```python
from build123d import *
from build123d.topology import SkipClean

# Parameters (mm, degrees)
SKETCH1_R                = 17.928932
BOSS_EXTRUDE1_DEPTH      = 10
SKETCH2_R                = 7.928932
CUT_EXTRUDE1_DEPTH       = 28.256068
BOSS_EXTRUDE2_REACH      = 46.834
BOSS_EXTRUDE2_END_RADIUS = 17.928932
SKETCH4_R                = 5
BOSS_EXTRUDE5_REACH      = 48.578
BOSS_EXTRUDE5_END_RADIUS = 17.928932
SKETCH11_R               = 5
CUT_EXTRUDE5_DEPTH       = 4
CIRPATTERN1_COUNT        = 2
CIRPATTERN1_ANGLE        = 270
SKETCH21_R               = 7.928932
BOSS_EXTRUDE6_DEPTH      = 20
SKETCH22_R               = 7.928932
BOSS_EXTRUDE7_DEPTH      = 20


with BuildPart() as part:
    # Sketch1 → Boss-Extrude1 (new body)
    with BuildSketch(Plane(origin=(0, 0, 0), x_dir=(1, 0, 0), z_dir=(0, 1, 0))):
        with Locations(Location((0, 0, 0), (0, 0, 270))):
            Circle(SKETCH1_R)
    extrude(amount=BOSS_EXTRUDE1_DEPTH)

    # Sketch2 → Cut-Extrude1 (cut, through all)
    with BuildSketch(Plane(origin=(0, 10, 0), x_dir=(1, 0, 0), z_dir=(0, 1, 0))):
        with Locations(Location((0, 0, 0), (0, 0, 270))):
            Circle(SKETCH2_R)
    extrude(amount=-CUT_EXTRUDE1_DEPTH, mode=Mode.SUBTRACT)

    # Boss-Extrude2: up to this cylinder (the profile starts outside it)
    with SkipClean():  # the faces are left unmerged after this step: merging them gives an invalid solid
        boss_extrude2_end = Plane(origin=(0, 5, 0), z_dir=(0, -1, 0)) * Cylinder(BOSS_EXTRUDE2_END_RADIUS, 130.525864, mode=Mode.PRIVATE)
        # Sketch4 → Boss-Extrude2 (add, up to the surface)
        with BuildSketch(Plane(origin=(21.928932, 0, 0), x_dir=(0, 0, -1), z_dir=(1, 0, 0)), mode=Mode.PRIVATE) as boss_extrude2_sk1:
            with Locations((0, 5)):
                Circle(SKETCH4_R)
        boss_extrude2_tool1 = extrude(boss_extrude2_sk1.sketch, amount=-BOSS_EXTRUDE2_REACH, mode=Mode.PRIVATE) - boss_extrude2_end
        add(boss_extrude2_tool1.solids().sort_by_distance((21.928932, 5, 0))[0])

    # Boss-Extrude5: up to this cylinder (the profile starts outside it)
    boss_extrude5_end = Plane(origin=(0, 5, 0), z_dir=(0, -1, 0)) * Cylinder(BOSS_EXTRUDE5_END_RADIUS, 134.013864, mode=Mode.PRIVATE)
    # Sketch11 → Boss-Extrude5 (add, up to the surface)
    with BuildSketch(Plane.XY.offset(-21.928932), mode=Mode.PRIVATE) as boss_extrude5_sk1:
        with Locations(Location((0, 5, 0), (0, 0, 270))):
            Circle(SKETCH11_R)
    boss_extrude5_tool1 = extrude(boss_extrude5_sk1.sketch, amount=BOSS_EXTRUDE5_REACH, mode=Mode.PRIVATE) - boss_extrude5_end
    add(boss_extrude5_tool1.solids().sort_by_distance((0, 5, -21.928932))[0])

    # Sketch14 → Cut-Extrude5 (cut)
    with BuildSketch(Plane(origin=(0, 0, -21.928932), x_dir=(-1, 0, 0), z_dir=(0, 0, -1))):
        Polygon((0, 8), (-0.33838, 7.678553), (-0.74607, 7.905749), (-0.993878, 7.510249), (-1.445261, 7.62892), (-1.586927, 7.184218), (-2.053641, 7.186906), (-2.080264, 6.720944), (-2.532984, 6.60748), (-2.44289, 6.149537), (-2.85317, 5.927051), (-2.65202, 5.5059), (-2.99408, 5.188372), (-2.694514, 4.830476), (-2.946862, 4.437856), (-2.567702, 4.165703), (-2.714481, 3.722662), (-2.279552, 3.553353), (-2.31154, 3.087728), (-1.848169, 3.0319), (-1.763356, 2.572949), (-1.300659, 2.634111), (-1.104374, 2.210671), (-0.671423, 2.384979), (-0.376, 2.023656), (0, 2.300158), (0.376, 2.023656), (0.671423, 2.384979), (1.104374, 2.210671), (1.300659, 2.634111), (1.763356, 2.572949), (1.848169, 3.0319), (2.31154, 3.087728), (2.279552, 3.553353), (2.714481, 3.722662), (2.567702, 4.165703), (2.946862, 4.437856), (2.694514, 4.830476), (2.99408, 5.188372), (2.65202, 5.5059), (2.85317, 5.927051), (2.44289, 6.149537), (2.532984, 6.60748), (2.080264, 6.720944), (2.053641, 7.186906), (1.586927, 7.184218), (1.445261, 7.62892), (0.993878, 7.510249), (0.74607, 7.905749), (0.33838, 7.678553), align=None)
    cut_extrude5 = extrude(amount=-CUT_EXTRUDE5_DEPTH, mode=Mode.SUBTRACT)

    # CirPattern1: Cut-Extrude5 ×2 about axis
    cirpattern1_axis = Axis((0, 0, 0), (0, 1, 0))
    for i in range(1, CIRPATTERN1_COUNT):
        add(cut_extrude5.rotate(cirpattern1_axis, i * CIRPATTERN1_ANGLE / (CIRPATTERN1_COUNT - 1)), mode=Mode.SUBTRACT)

    # Sketch21 → Boss-Extrude6 (add)
    with BuildSketch(Plane(origin=(0, 10, 0), x_dir=(1, 0, 0), z_dir=(0, 1, 0))):
        with BuildLine():
            ThreePointArc((17.928932, 0), (12.67767, 12.67767), (0, 17.928932))
            ThreePointArc((0, 17.928932), (-12.67767, -12.67767), (17.928932, 0))
        make_face()
        with Locations(Location((0, 0, 0), (0, 0, 270))):
            Circle(SKETCH21_R, mode=Mode.SUBTRACT)
    extrude(amount=BOSS_EXTRUDE6_DEPTH)

    # Sketch22 → Boss-Extrude7 (add)
    with BuildSketch(Plane.XZ):
        with BuildLine():
            ThreePointArc((0, -17.928932), (12.67767, -12.67767), (17.928932, 0))
            ThreePointArc((17.928932, 0), (-12.67767, 12.67767), (0, -17.928932))
        make_face()
        with Locations(Location((0, 0, 0), (0, 0, 90))):
            Circle(SKETCH22_R, mode=Mode.SUBTRACT)
    extrude(amount=BOSS_EXTRUDE7_DEPTH)


solid = part.part
```
The model under review builds one solid part; all positions refer to its coordinate system, in mm. A direction names the side the tool comes from. Coordinates: 2 decimals unless noted, no trailing zeros. Write each loop counter-clockwise with the first axis right and the second up, starting at its lowest first coordinate (ties: lowest second). Pieces come first, ordered by that corner, then holes.
1) We need section C-C on z = -11. State the section outline as (x, y) points.
2) We need section A-A on x = 6.5. State the section outline as (y, z) points, then the cut area to 3 significant figures.
3) To check wall thickness, follow probe 1 along Z at (x, y) = (0, 3); probe 2 along X at (y, z) = (2, 0). State the ranges of each line that lie inside material, in increasing order.
4) The part is to be moulded in two halves that separate along Y. For faces 3 (the face through (-2.2, 2.8, -21.929)), 4 (the face through (0, 5, -17.929)), 5 (the face through (1.5, 0.23, -19.61)), say which applies: pulls with the +Y half, pulls with the -Y half, needs draft (parallel to the pull), parting line crosses it, or undercut.
5) Machinability: for faces 1 (the face through (4, -20, -8)), 2 (the face through (19.61, 0.12, 1.08)), which of the approach directions +Z, -Z, +X, -X, +Y, -Y give a long, thin tool a straight path to every point of the face, cutting with its end or side? Answer none if there is none.
6) Clearance check with flat-ended pins moving along their axes: pin 1 Ø8 at (y, z) = (4, -4.5) entering from -X; pin 2 Ø3 at (x, y) = (12, -1.5) entering from -Z; pin 3 Ø12 at (x, y) = (0, -12.5) entering from -Z. State where each tip first meets the part, or that it passes through.
7) We need section D-D on z = 10.5. State the section outline as (x, y) points, then the cut area to 3 significant figures.
8) We need section B-B on y = -13. State the section outline as (x, z) points, then the cut area to 3 significant figures.
Answer list:
1. outline: (-14.16, -20) - (14.16, -20) - (14.16, 30) - (-14.16, 30) - close
2. outline: (-20, -16.71) - (30, -16.71) - (30, -4.54) - (-20, -4.54) - close; (-20, 4.54) - (30, 4.54) - (30, 16.71) - (-20, 16.71) - close
2. area: 1,220 mm2
3. probe 1: z = -17.93 to -7.93, 7.93 to 17.93
3. probe 2: x = -17.93 to -7.93, 7.93 to 21.93
4. face 3: needs draft
4. face 4: undercut
4. face 5: parting line crosses it
5. face 1: +Z, -Z, +X, -X, -Y
5. face 2: +X
6. pin 1: stops at x = -17.92
6. pin 2: stops at z = -14.53
6. pin 3: stops at z = -17.93
7. outline: (-14.53, -20) - (14.53, -20) - (14.53, 30) - (-14.53, 30) - close
7. area: 1,450 mm2
8. outline: (0, -17.93) arc R17.93 ccw to (17.93, 0) arc R17.93 ccw (long way) to start; hole circle Ø15.86 at (0, 0)
8. area: 812 mm2
